Part model, mm, in its own coordinate system. A direction names the side the tool comes from. Round coordinates to 2 decimals unless told otherwise and drop trailing zeros. Loops run counter-clockwise (first coordinate to the right, second up) from the corner with the lowest first, then second, coordinate; pieces in that order, holes last. Notation, with made-up numbers: (17.25, -39) - (22.25, -39) arc R33 cw to (22.25, -8) - close; hole circle Ø7 at (58.5, 86). An arc over 180 degrees is marked (long way). Write each question's results on one line, items separated by ' | '. Start each with the question number.
(1) Flat gauge pins, fed straight in: P1, Ø1, axis at y = -22.5, z = 2.5, coming from the -X side; P2, Ø3, axis at x = -31.47, y = -31.47, coming from the +Z side. Where does each tip first touch, or does it go through?
(2) Cut at A-A, the plane y = 0. List the corners of the cut face in (x, z), then the cut area to 3 significant figures.
(3) Mould opens along X. For faces 3 (the face through (-2.57, 47.18, 1.48)), 4 (the face through (-34, -3, 0)), 5 (the face through (-0.412, 42.645, 1.479)) say: released by +X, released by -X, zero draft, split by the parting line, or undercut.
(4) Cut at C-C, the plane z = 0.6. List the corners of the cut face in (x, y) (3 decimals).
(5) Cut at B-B, the plane x = 0. List the corners of the cut face in (y, z), then the cut area to 3 significant figures.
(6) Cut at D-D, the plane y = 26.5. List the corners of the cut face in (x, z).
(7) Drill centre lines: L1, parallel to Y at x = 0, z = 1.05; L2, parallel to Y at x = -48, z = 2.35; L3, parallel to Y at x = 30.5, z = 1.75. Where is each one in solid material? Low to high.
(8) Tool access for faces 1 (the face through (-50, 19.95, 2)), 2 (the face through (-34, -3, 3)): list every direction of +Z, -Z, +X, -X, +Y, -Y with a clear straight run to the whole face (end or side of a thin tool).
from build123d import *

# Parameters (mm, degrees)
SKETCH_1_R          = 47.25
SKETCH_1_R_2        = 1.9
SKETCH_1_R_3        = 32.5
EXTRUDE_1_DEPTH     = 3
CUT_EXTRUDE_START   = -3
CUT_EXTRUDE_1_DEPTH = 3
EXTRUDE_2_DEPTH     = 3
FILLET_1_R          = 3
FILLET_2_R          = 6


with BuildPart() as part:
    # 草图1 → 凸台-拉伸1 (new body)
    with BuildSketch(Plane.XY):
        Circle(SKETCH_1_R)
        with Locations((-31.466251763, -31.466251763)):
            Circle(SKETCH_1_R_2, mode=Mode.SUBTRACT)
        with Locations((-42.5, 0)):
            Circle(SKETCH_1_R_2, mode=Mode.SUBTRACT)
        Circle(SKETCH_1_R_3, mode=Mode.SUBTRACT)
        with Locations((0, -44.5)):
            Circle(SKETCH_1_R_2, mode=Mode.SUBTRACT)
        with Locations((31.466251763, -31.466251763)):
            Circle(SKETCH_1_R_2, mode=Mode.SUBTRACT)
        with Locations((-31.466251763, 31.466251763)):
            Circle(SKETCH_1_R_2, mode=Mode.SUBTRACT)
        with Locations((0, 44.5)):
            Circle(SKETCH_1_R_2, mode=Mode.SUBTRACT)
        with Locations((42.5, 0)):
            Circle(SKETCH_1_R_2, mode=Mode.SUBTRACT)
        with Locations((31.466251763, 31.466251763)):
            Circle(SKETCH_1_R_2, mode=Mode.SUBTRACT)
    extrude(amount=EXTRUDE_1_DEPTH)

    # 草图2 → 切除-拉伸1 (cut)
    with BuildSketch(Plane.XY.offset(3).offset(CUT_EXTRUDE_START)):
        with BuildLine():
            ThreePointArc((40.6, 0), (42.5, 1.9), (44.4, 0))
            Line((44.4, 0), (47.25, 0))
            ThreePointArc((47.25, 0), (44.807674543, 14.994492391), (37.733182981, 28.438871323))
            ThreePointArc((37.733182981, 28.438871323), (38.837402493, 26.340410113), (39.218611997, 24))
            ThreePointArc((39.218611997, 24), (34.184022114, 17.006209505), (25.954041018, 19.561128669))
            ThreePointArc((25.954041018, 19.561128669), (30.820093552, 10.313672161), (32.5, 0))
            Line((32.5, 0), (40.6, 0))
        make_face()
        with BuildLine():
            Line((47.25, 0), (44.4, 0))
            ThreePointArc((44.4, 0), (42.5, -1.9), (40.6, 0))
            Line((40.6, 0), (32.5, 0))
            ThreePointArc((32.5, 0), (30.820093563, -10.313672127), (25.954041062, -19.561128611))
            ThreePointArc((25.954041062, -19.561128611), (34.184022149, -17.006209517), (39.218611997, -24))
            ThreePointArc((39.218611997, -24), (38.837402455, -26.340410225), (37.733182838, -28.438871512))
            ThreePointArc((37.733182838, -28.438871512), (44.807674505, -14.994492504), (47.25, 0))
        make_face()
    extrude(amount=CUT_EXTRUDE_1_DEPTH, mode=Mode.SUBTRACT)


with BuildPart() as cut_extrude_1_kept_piece:
    # of the separate pieces the step leaves, the one the design keeps (cut_extrude_1_pieces_kept)
    add(part.part.solids().sort_by_distance((-29.566251763, -31.466251763, 3))[0])

    # 草图3 → 凸台-拉伸2 (add)
    with BuildSketch(Plane.XY.offset(3)):
        with BuildLine():
            Line((-42.831763914, 19.95), (-56.831763914, 19.95))
            Line((-56.831763914, 19.95), (-56.831763914, 0))
            Line((-56.831763914, 0), (-47.25, 0))
            ThreePointArc((-47.25, 0), (-46.132219462, 10.216693571), (-42.831763914, 19.95))
        make_face()
        with BuildLine():
            Line((-47.25, 0), (-56.831763914, 0))
            Line((-56.831763914, 0), (-56.831763914, -19.95))
            Line((-56.831763914, -19.95), (-42.831763914, -19.95))
            ThreePointArc((-42.831763914, -19.95), (-46.132219462, -10.216693571), (-47.25, 0))
        make_face()
    extrude(amount=-EXTRUDE_2_DEPTH)

    # 圆角1
    fillet_1_edges = [cut_extrude_1_kept_piece.edges().sort_by_distance(p)[0] for p in [
        (-56.831763914, -19.95, 1.5),
        (-56.831763914, 19.95, 1.5),
    ]]
    fillet(fillet_1_edges, radius=FILLET_1_R)

    # 圆角2
    fillet_2_edges = [cut_extrude_1_kept_piece.edges().sort_by_distance(p)[0] for p in [
        (-42.831763914, 19.95, 1.5),
        (-42.831763914, -19.95, 1.5),
    ]]
    fillet(fillet_2_edges, radius=FILLET_2_R)


solid = cut_extrude_1_kept_piece.part
A:
1) P1: x = -41.98 | P2: through
2) outline: (-56.83, 0) - (-44.4, 0) - (-44.4, 3) - (-56.83, 3) - close; (-40.6, 0) - (-32.5, 0) - (-32.5, 3) - (-40.6, 3) - close | area: 61.6 mm2
3) face 3: split by the parting line | face 4: zero draft | face 5: undercut
4) outline: (-56.832, -16.95) arc R3 ccw to (-53.832, -19.95) - (-46.499, -19.95) arc R6 cw to (-41.26, -23.026) arc R47.25 ccw to (37.733, -28.439) arc R7.375 ccw to (25.954, -19.561) arc R32.5 cw (long way) to (25.954, 19.561) arc R7.375 ccw to (37.733, 28.439) arc R47.25 ccw to (-41.26, 23.026) arc R6 cw to (-46.499, 19.95) - (-53.832, 19.95) arc R3 ccw to (-56.832, 16.95) - close; hole circle Ø3.8 at (-42.5, 0); hole circle Ø3.8 at (-31.466, -31.466); hole circle Ø3.8 at (-31.466, 31.466); hole circle Ø3.8 at (0, -44.5); hole circle Ø3.8 at (0, 44.5); hole circle Ø3.8 at (31.466, -31.466); hole circle Ø3.8 at (31.466, 31.466)
5) outline: (-47.25, 0) - (-46.4, 0) - (-46.4, 3) - (-47.25, 3) - close; (-42.6, 0) - (-32.5, 0) - (-32.5, 3) - (-42.6, 3) - close; (32.5, 0) - (42.6, 0) - (42.6, 3) - (32.5, 3) - close; (46.4, 0) - (47.25, 0) - (47.25, 3) - (46.4, 3) - close | area: 65.7 mm2
6) outline: (-39.12, 0) - (-18.81, 0) - (-18.81, 3) - (-39.12, 3) - close; (18.81, 0) - (38.78, 0) - (38.78, 3) - (18.81, 3) - close
7) L1: -47.25 to -46.4, -42.6 to -32.5, 32.5 to 42.6, 46.4 to 47.25 | L2: -19.95 to 19.95 | L3: -36.09 to -33.1, -29.83 to -16.75, 16.75 to 29.83, 33.1 to 36.09
8) face 1: +Z, -Z, -X, +Y | face 2: +Z, +X, -X, +Y, -Y
